Read the model definition and answer for the solid it produces. Units are mm, in the model's axes. A direction names the side the tool comes from. Give positions to 0.01 mm unless a question says otherwise; leave off trailing zeros. Use a Markdown table: item, result. Add a question column.
1. Flat-ended cylindrical pins translate along their axes: P1, Ø15, axis at y = 691, z = -97.5, coming from the -X side; P2, Ø14, axis at y = 397, z = -89, coming from the +X side; P3, Ø4, axis at y = 260.5, z = 24, coming from the +X side. Find the tip coordinate at first contact, or state that the pin passes through.
2. Consider L1, parallel to Y at x = -190, z = -80; L2, parallel to Y at x = 193, z = -33; L3, parallel to X at y = 701.5, z = 20. Determine where each line is inside the solid, lowest interval first.
3. Which of the six approach directions +Z, -Z, +X, -X, +Y, -Y give full straight-line access (tool end or side, diameter ignored) to faces 1 (the flat face through (193, 429.557, -74)), 2 (the flat face through (-253.777, 700, -74)), 3 (the flat face through (100.263, 406, -74)), 4 (the flat face through (15, 735, -74))?
4. For a pull along Z with two mould halves and no side action, classify faces 5 (the flat face through (-71, 155, -133)), 6 (the flat face through (8, 700, -140)), 7 (the flat face through (353, 347, 15)) as released by +Z, released by -Z, zero draft, split by the parting line, or undercut.
5. A cutting plane is placed at A-A on z = -58.5. State how many separate pieces and enclosed holes the cut face has, and give its area (3 significant figures).
```python
from build123d import *

# Parameters (mm, degrees)
CORTE_EXTRUS_O3_REACH     = 1164.591
ESBO_O5_R                 = 5
CORTE_EXTRUS_O4_DEPTH     = 10
ESBO_O8_W                 = 680
ESBO_O8_H                 = 1040
RESSALTO_EXTRUS_O1_DEPTH  = 20
FILETE1_R                 = 10
ESBO_O11_W                = 22.5
ESBO_O11_H                = 480
CORTE_EXTRUS_O5_DEPTH     = 35
CORTE_EXTRUS_O6_DEPTH     = 35
FILETE15_R                = 10
RESSALTO_EXTRUS_O2_DEPTH  = 120
FILETE16_R                = 10
RESSALTO_EXTRUS_O4_DEPTH  = 120
ESBO_O16_W                = 319.937855213
ESBO_O16_H                = 10
RESSALTO_EXTRUS_O5_DEPTH  = 36.138
FILETE17_R                = 10
RESSALTO_EXTRUS_O6_DEPTH  = 120
ESBO_O18_W                = 162.736994832
ESBO_O18_H                = 10
RESSALTO_EXTRUS_O7_DEPTH  = 46.138
FILETE18_R                = 10
ESBO_O19_W                = 531.126065259
ESBO_O19_H                = 10
RESSALTO_EXTRUS_O8_DEPTH  = 120
RESSALTO_EXTRUS_O9_DEPTH  = 50
FILETE19_R                = 10
ESBO_O22_W                = 529.518507703
ESBO_O22_H                = 10
RESSALTO_EXTRUS_O10_DEPTH = 35


with BuildPart() as part:
    # Esboço2 for Loft1 → Loft1 section 0
    with BuildSketch(Plane(origin=(0, 1100, 0), x_dir=(1, 0, 0), z_dir=(0, 1, 0))):
        with BuildLine():
            Line((-370, 0), (370, 0))
            Line((370, 0), (370, -40))
            # circular arc as an exact rational Bezier (weights 1, cos(half-angle), 1)
            Bezier((370, -40), (0, -97.731859317), (-370, -40), weights=[1, 0.988044857, 1])
            Line((-370, -40), (-370, 0))
        make_face()
    # Esboço1 for Loft1 → Loft1 section 1
    with BuildSketch(Plane(origin=(0, 0, 0), x_dir=(1, 0, 0), z_dir=(0, 1, 0))):
        with BuildLine():
            Line((-370, 0), (370, 0))
            Line((370, 0), (370, -50))
            Bezier((370, -50), (0, -82.722461177), (-370, -50), weights=[1, 0.996112056, 1])
            Line((-370, -50), (-370, 0))
        make_face()
    loft()

    # Esboço5 → Corte-extrusão3 (cut, up to next)
    with BuildSketch(Plane.XZ, mode=Mode.PRIVATE) as corte_extrus_o3_sk1:
        with Locations(Location((-350, 20, 0), (0, 0, 270))):
            Circle(ESBO_O5_R)
    corte_extrus_o3_tool1 = extrude(corte_extrus_o3_sk1.sketch, amount=-CORTE_EXTRUS_O3_REACH, mode=Mode.PRIVATE) & part.part
    add(corte_extrus_o3_tool1.solids().sort_by_distance((-350, 0, 20))[0], mode=Mode.SUBTRACT)

    # Esboço6 → Corte-extrusão4 (cut)
    with BuildSketch(Plane.XZ):
        with BuildLine():
            Line((-370, 0), (-320.856761827, 0))
            Line((-320.856761827, 0), (-320.856761827, 10.441916975))
            ThreePointArc((-320.856761827, 10.441916975), (-325.250160109, 21.048518693), (-335.856761827, 25.441916975))
            Line((-335.856761827, 25.441916975), (-370, 25.441916975))
            Line((-370, 25.441916975), (-370, 0))
        make_face()
    extrude(amount=-CORTE_EXTRUS_O4_DEPTH, mode=Mode.SUBTRACT)

    # Esboço8 → Ressalto-extrusão1 (add)
    with BuildSketch(Plane(origin=(0, 0, 0), x_dir=(-1, 0, 0), z_dir=(0, 0, -1))):
        with Locations((-5, 555)):
            Rectangle(ESBO_O8_W, ESBO_O8_H)
    extrude(amount=RESSALTO_EXTRUS_O1_DEPTH)

    # Filete1
    filete1_edges = [part.edges().sort_by_distance(p)[0] for p in [
        (-335, 555, 0),
        (-335, 35, -10),
        (5, 1075, 0),
        (-335, 1075, -10),
        (345, 555, 0),
        (345, 1075, -10),
        (5, 35, 0),
        (345, 35, -10),
        (-335, 555, -20),
        (345, 555, -20),
        (5, 35, -20),
    ]]
    fillet(filete1_edges, radius=FILETE1_R - 0.0001)  # a hair under: the kernel refuses the full size

    # Esboço11 → Corte-extrusão5 (cut)
    with BuildSketch(Plane(origin=(370, 0, 0), x_dir=(0, 0, -1), z_dir=(1, 0, 0))):
        with Locations((-26.25, 350)):
            Rectangle(ESBO_O11_W, ESBO_O11_H)
    extrude(amount=-CORTE_EXTRUS_O5_DEPTH, mode=Mode.SUBTRACT)

    # Esboço12 → Corte-extrusão6 (cut)
    with BuildSketch(Plane(origin=(370, 0, 0), x_dir=(0, 0, -1), z_dir=(1, 0, 0))):
        with BuildLine():
            Line((-15, 110), (-37.5, 110))
            ThreePointArc((-37.5, 110), (-26.25, 102.175823272), (-15, 110))
        make_face()
        with BuildLine():
            Line((-15, 590), (-37.5, 590))
            ThreePointArc((-37.5, 590), (-26.25, 597.824176728), (-15, 590))
        make_face()
    extrude(amount=-CORTE_EXTRUS_O6_DEPTH, mode=Mode.SUBTRACT)

    # Filete15
    filete15_edges = [part.edges().sort_by_distance(p)[0] for p in [
        (335, 350, 37.5),
    ]]
    fillet(filete15_edges, radius=FILETE15_R)

    # Esboço13 → Ressalto-extrusão2 (add)
    with BuildSketch(Plane(origin=(0, 0, -20), x_dir=(-1, 0, 0), z_dir=(0, 0, -1))):
        Polygon((260, 155), (250, 155), (250, 190), (-280, 190), (-280, 155), (-290, 155), (-290, 200), (260, 200), align=None)
    extrude(amount=RESSALTO_EXTRUS_O2_DEPTH)

    # Filete16
    filete16_edges = [part.edges().sort_by_distance(p)[0] for p in [
        (290, 200, -80),
        (-260, 200, -80),
        (15, 200, -140),
        (-260, 177.5, -140),
        (290, 177.5, -140),
    ]]
    fillet(filete16_edges, radius=FILETE16_R - 0.0001)  # a hair under: the kernel refuses the full size

    # Esboço15 → Ressalto-extrusão4 (add)
    with BuildSketch(Plane(origin=(0, 0, -20), x_dir=(-1, 0, 0), z_dir=(0, 0, -1))):
        Polygon((253.776635588, 383.41937577), (243.776635588, 383.41937577), (243.776635588, 419.557368326), (-76.161219625, 419.557368326), (-76.161219625, 383.41937577), (-86.161219625, 383.41937577), (-86.161219625, 429.557368326), (253.776635588, 429.557368326), align=None)
    extrude(amount=RESSALTO_EXTRUS_O4_DEPTH)

    # Esboço16 → Ressalto-extrusão5 (add)
    with BuildSketch(Plane.XZ.offset(-419.557368326)):
        with Locations((-83.807707982, -135)):
            Rectangle(ESBO_O16_W, ESBO_O16_H)
    extrude(amount=RESSALTO_EXTRUS_O5_DEPTH)

    # Filete17
    filete17_edges = [part.edges().sort_by_distance(p)[0] for p in [
        (-253.776635588, 429.557368326, -80),
        (86.161219625, 429.557368326, -80),
        (-253.776635588, 406.488372048, -140),
        (-83.807707982, 429.557368326, -140),
        (86.161219625, 406.488372048, -140),
    ]]
    fillet(filete17_edges, radius=FILETE17_R - 0.0001)  # a hair under: the kernel refuses the full size

    # Esboço17 → Ressalto-extrusão6 (add)
    with BuildSketch(Plane(origin=(0, 0, -20), x_dir=(-1, 0, 0), z_dir=(0, 0, -1))):
        Polygon((-100.263005168, 439.557368326), (-283, 439.557368326), (-283, 383.41937577), (-273, 383.41937577), (-273, 429.557368326), (-110.263005168, 429.557368326), (-110.263005168, 383.41937577), (-100.263005168, 383.41937577), align=None)
    extrude(amount=RESSALTO_EXTRUS_O6_DEPTH)

    # Esboço18 → Ressalto-extrusão7 (add)
    with BuildSketch(Plane(origin=(0, 429.557368326, 0), x_dir=(-1, 0, 0), z_dir=(0, -1, 0))):
        with Locations((-191.631502584, 135)):
            Rectangle(ESBO_O18_W, ESBO_O18_H)
    extrude(amount=RESSALTO_EXTRUS_O7_DEPTH)

    # Filete18
    filete18_edges = [part.edges().sort_by_distance(p)[0] for p in [
        (100.263005168, 439.557368326, -80),
        (283, 439.557368326, -80),
        (100.263005168, 411.488372048, -140),
        (191.631502584, 439.557368326, -140),
        (283, 411.488372048, -140),
    ]]
    fillet(filete18_edges, radius=FILETE18_R - 0.0001)  # a hair under: the kernel refuses the full size

    # Esboço19 → Ressalto-extrusão8 (add)
    with BuildSketch(Plane(origin=(0, 0, -20), x_dir=(-1, 0, 0), z_dir=(0, 0, -1))):
        with Locations((-11.786397041, 730)):
            Rectangle(ESBO_O19_W, ESBO_O19_H)
    extrude(amount=RESSALTO_EXTRUS_O8_DEPTH)

    # Esboço20 → Ressalto-extrusão9 (add)
    with BuildSketch(Plane.XZ.offset(-725)):
        Polygon((-253.776635588, -20), (-253.776635588, -140), (277.349429671, -140), (277.349429671, -20), (267.349429671, -20), (267.349429671, -130), (-243.776635588, -130), (-243.776635588, -20), align=None)
    extrude(amount=RESSALTO_EXTRUS_O9_DEPTH)

    # Filete19
    filete19_edges = [part.edges().sort_by_distance(p)[0] for p in [
        (277.349429671, 735, -80),
        (-253.776635588, 735, -80),
        (277.349429671, 705, -140),
        (-253.776635588, 705, -140),
        (11.786397041, 735, -140),
    ]]
    fillet(filete19_edges, radius=FILETE19_R)

    # Esboço22 → Ressalto-extrusão10 (add)
    with BuildSketch(Plane.XZ.offset(-190)):
        with Locations((14.759253851, -135)):
            Rectangle(ESBO_O22_W, ESBO_O22_H)
    extrude(amount=RESSALTO_EXTRUS_O10_DEPTH)


solid = part.part
```
Output values:
| question | item | result |
|---|---|---|
| 1 | P1 | x = -253.78 |
| 1 | P2 | x = 283 |
| 1 | P3 | x = 335 |
| 2 | L1 | 190 to 200, 419.56 to 429.56, 725 to 735 |
| 2 | L2 | 190 to 200, 429.56 to 439.56, 725 to 735 |
| 2 | L3 | -370 to -355, -345 to 370 |
| 3 | face 1 | none |
| 3 | face 2 | -Z, -X, +Y |
| 3 | face 3 | -Z |
| 3 | face 4 | -Z, +X, -X, +Y |
| 4 | face 5 | zero draft |
| 4 | face 6 | released by -Z |
| 4 | face 7 | undercut |
| 5 | separate pieces | 4 |
| 5 | enclosed holes | 0 |
| 5 | area | 19,200 mm² |
